Source: three-view drawing plus pictorial views. Frame: mm from the lowest corner of the part. A direction names the side the tool comes from. Round coordinates to 2 decimals unless told otherwise and drop trailing zeros. Write each loop counter-clockwise with the first axis right and the second up, starting at its lowest first coordinate (ties: lowest second). Pieces come first, ordered by that corner, then holes. Notation, with made-up numbers: M 63.5,-11.5 L 104.5,-11.5 A13 ccw 104.5,-3.5 Z; hole C 70.5,60 d3. An arc over 180 degrees is marked long. Answer as CSV lines item,"result". Start each with the question number.
Q1. Section query B-B on z = 65. Output: boundary loops of the cut face in (x, y).
Q2. Section query A-A on x = 65. Output: boundary loops of the cut face in (y, z).
Q3. First-contact query: pin 1 (1.5 mm diameter, centred on x = 72.5, y = 43, fed in from +Z); pin 2 (10 mm diameter, centred on y = 25.5, z = 50.5, fed in from -X); pin 3 (6 mm diameter, centred on y = 90.5, z = 37.5, fed in from -X). Flat tips, straight axial feed; report the tip coordinate or a pass-through.
Q4. Reachability of the marked faces 5, 6 and 7 from +Z, -Z, +X, -X, +Y, -Y: full face, straight path, thin tool, end or side. Return the list, or none.
Q5. Ray query, probe 1 along Z at (x, y) = (65, 93.5); probe 2 along Z at (x, y) = (107, 104); probe 3 along X at (y, z) = (52, 15.5) (1 decimal). Return the intervals inside material, ascending.
Q6. Mould query, pull axis Z, two halves, no side actions, for the marked faces 1, 2, 3 and 4. Classes: pulls with the +Z half, pulls with the -Z half, needs draft (parallel to the pull), parting line crosses it, or undercut.
Q7. Section query C-C on y = 78. Output: boundary loops of the cut face in (x, z), and give its area (3 significant figures).
Q8. Section query D-D on y = 50. Output: boundary loops of the cut face in (x, z), and give its area (3 significant figures).
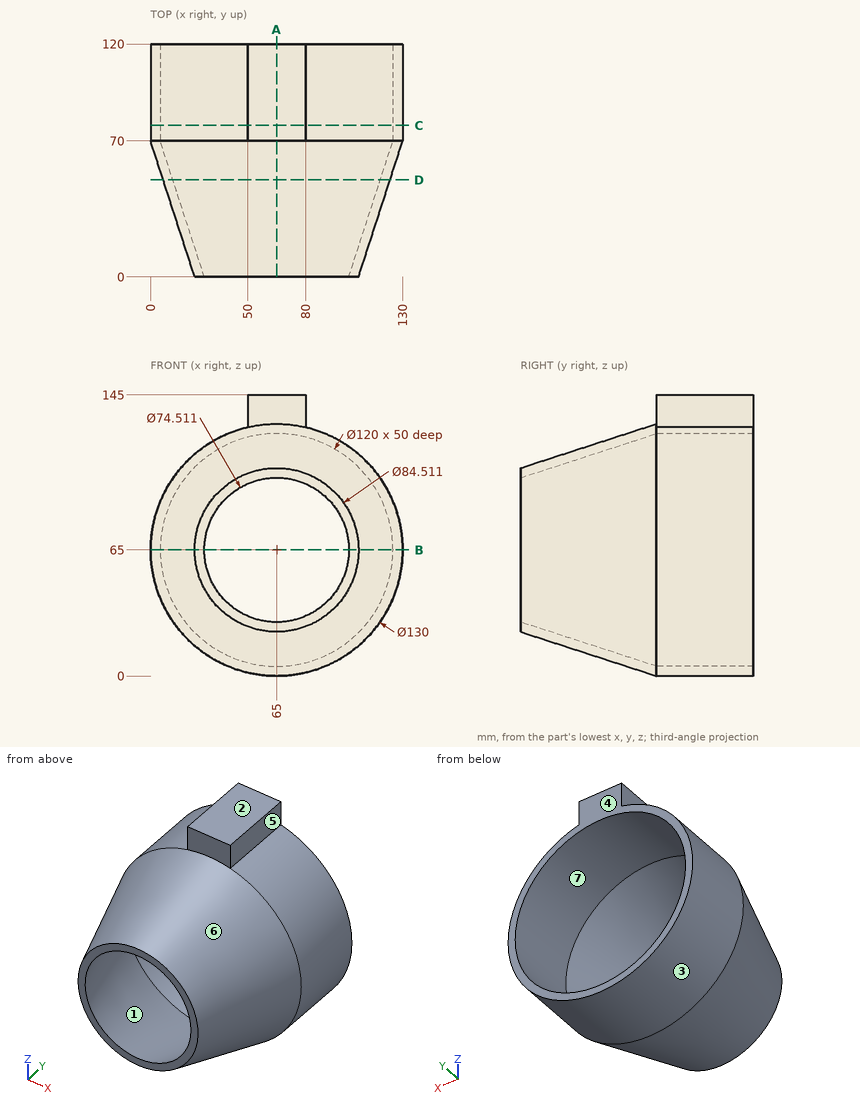
Entries:
1,outline,"M 0,70 L 22.74,0 L 27.74,0 L 5,70 L 5,120 L 0,120 Z; M 102.26,0 L 107.26,0 L 130,70 L 130,120 L 125,120 L 125,70 Z"
2,outline,"M 0,22.74 L 70,0 L 120,0 L 120,5 L 70,5 L 0,27.74 Z; M 0,102.26 L 70,125 L 120,125 L 120,145 L 70,145 L 70,130 L 0,107.26 Z"
3,pin 1,"stops at z = 120.99"
3,pin 2,"stops at x = 14.45"
3,pin 3,"stops at x = 4.79"
4,face 5,"+Z, +X, +Y, -Y"
4,face 6,"-Y"
4,face 7,"+Y"
5,probe 1,"z = 0 to 5, 125 to 145"
5,probe 2,"z = 15.39 to 22.15, 107.85 to 114.61"
5,probe 3,"x = 32.6 to 43, 87 to 97.4"
6,face 1,"undercut"
6,face 2,"pulls with the +Z half"
6,face 3,"parting line crosses it"
6,face 4,"needs draft"
7,outline,"M 50,128.25 A65 ccw long 80,128.25 L 80,145 L 50,145 Z; hole C 65,65 d120"
7,area,"2,430 mm^2"
8,outline,"C 65,65 d117; hole C 65,65 d107"
8,area,"1,760 mm^2"
